Could you check a few things on this model? Use its own coordinates, in mm. A direction names the side the tool comes from. Give positions to 0.01 mm unless a question says otherwise; leave off trailing zeros. Order: outer loops, then holes, each group sorted by start corner. A loop starts at its lowest first (then second) coordinate and runs counter-clockwise, first axis right, second up. Notation, with made-up numbers: M 34,5.25 L 40,5.25 A9 ccw 40,11.25 Z; hole C 43,82.25 d8. An arc over 180 degrees is marked long. Answer in a Markdown table with one row per item. Add a question column.
```python
from build123d import *

# Parameters (mm, degrees)
F0_W         = 4.5
F0_H         = 70
F0_W_2       = 4
F0_H_2       = 34
F1_DEPTH     = 5
F2_W         = 5
F2_H         = 10
F2_W_2       = 4
F2_H_2       = 5.5
F3_DEPTH     = 13
F4_R         = 2.1
F4_R_2       = 1
F5_DEPTH     = 28.001
F6_R         = 2.1
F7_DEPTH     = 3
F8_R         = 3.6
F8_R_2       = 2.1
F9_DEPTH     = 3.8
F10_R        = 7
F11_T1_DEPTH = 5


# Not quite as in the source:
# - a fillet or chamfer that OpenCascade refuses, or shapes differently, is made with other operations: its cross-section is extruded or revolved along the edge and cut away or added


with BuildPart() as f1:
    # F0 (on Front) → F1 (new body)
    with BuildSketch(Plane.XZ):
        Polygon((-8, -44), (8, -44), (8, 44), (-8, 44), (-8, 42), (-8, 8), align=None)
        Rectangle(F0_W, F0_H, mode=Mode.SUBTRACT)
        Polygon((-8, 44), (8, 44), (14, 44), (14, 54), (-14, 54), (-14, 44), align=None)
        with Locations((-10, 25)):
            Rectangle(F0_W_2, F0_H_2)
    extrude(amount=F1_DEPTH)

    # F2 (on face) → F3 (join)
    with BuildSketch(Plane.XZ.offset(5)):
        with Locations((11.5, 49)):
            Rectangle(F2_W, F2_H)
        with Locations((-11.5, 49)):
            Rectangle(F2_W, F2_H)
        with Locations((-10, 10.75)):
            Rectangle(F2_W_2, F2_H_2)
        with Locations((-10, 39.25)):
            Rectangle(F2_W_2, F2_H_2)
    extrude(amount=F3_DEPTH)

    # F4 (on face) → F5 (cut, through all)
    with BuildSketch(Plane(origin=(-14, 0, 0), x_dir=(0, -1, 0), z_dir=(-1, 0, 0))):
        with Locations((13, 49)):
            Circle(F4_R)
        with Locations((15.25, 39.25)):
            Circle(F4_R_2)
        with Locations((15.25, 10.75)):
            Circle(F4_R_2)
    extrude(amount=-F5_DEPTH, mode=Mode.SUBTRACT)

    # F6 (on face) → F7 (cut)
    with BuildSketch(Plane(origin=(-14, 0, 0), x_dir=(0, -1, 0), z_dir=(-1, 0, 0))):
        Polygon((15.0784609691, 45.4), (17.1569219382, 49), (15.0784609691, 52.6), (10.9215390309, 52.6), (8.8430780618, 49), (10.9215390309, 45.4), align=None)
        with Locations((13, 49)):
            Circle(F6_R, mode=Mode.SUBTRACT)
    extrude(amount=-F7_DEPTH, mode=Mode.SUBTRACT)

    # F8 (on face) → F9 (cut)
    with BuildSketch(Plane.YZ.offset(14)):
        with Locations((-13, 49)):
            Circle(F8_R)
        with Locations((-13, 49)):
            Circle(F8_R_2, mode=Mode.SUBTRACT)
    extrude(amount=-F9_DEPTH, mode=Mode.SUBTRACT)

    # F10
    f10_edges = [f1.edges().sort_by_distance(p)[0] for p in [
        (8, -2.5, -44),
        (-8, -2.5, -44),
    ]]
    fillet(f10_edges, radius=F10_R)

    # F11: fillet of radius 2.5 on 4 edges, made by hand

    # F11_s2 → F11_t1 (join)
    with BuildSketch(Plane.XZ):
        with BuildLine():
            ThreePointArc((0.25, -35), (-1.517766953, -34.267766953), (-2.25, -32.5))
            Line((-2.25, -32.5), (-2.25, -35))
            Line((-2.25, -35), (0.25, -35))
        make_face()
        with BuildLine():
            ThreePointArc((2.25, -32.5), (1.517766953, -34.267766953), (-0.25, -35))
            Line((-0.25, -35), (2.25, -35))
            Line((2.25, -35), (2.25, -32.5))
        make_face()
        with BuildLine():
            ThreePointArc((-2.25, 32.5), (-1.517766953, 34.267766953), (0.25, 35))
            Line((0.25, 35), (-2.25, 35))
            Line((-2.25, 35), (-2.25, 32.5))
        make_face()
        with BuildLine():
            ThreePointArc((2.25, 32.5), (1.517766953, 34.267766953), (-0.25, 35))
            Line((-0.25, 35), (2.25, 35))
            Line((2.25, 35), (2.25, 32.5))
        make_face()
    extrude(amount=F11_T1_DEPTH)


solid = f1.part
```
1. Suppose I cut it at C-C on z = 10.75. List the corners of the cut face in (x, y) for me, plus the area to 4 significant figures.
2. Suppose I cut it at D-D on x = 7. List the corners of the cut face in (y, z) for me.
3. If I drill on line 1 along X through (y, z) = (-1.5, 12.5); line 2 along Z through (x, y) = (9.6, -13); line 3 along Z through (x, y) = (11, -14), over which ranges is the centre line in solid material (lowest first)? Write a range as [from, to].
4. Thinking about a two-plate mould opening in Z: for faces 1 (the flat face through (9, -10, 49)), 2 (the cylindrical face through (-1.587, -2.465, -34.196)), 3 (the flat face through (-11, -9, 44)), 4 (the cylindrical face through (-6, -2.5, -41.9)), which applies, pulls with the +Z half, pulls with the -Z half, needs draft (parallel to the pull), parting line crosses it, or undercut?
5. Will these pins go through, and if not, where does the flat tip stop? P1, Ø1, axis at y = -5, z = -0.5, coming from the +X side; P2, Ø1.5, axis at y = -2.5, z = 2, coming from the -X side; P3, Ø4.5, axis at y = -11.5, z = 40, coming from the +X side.
6. Suppose I cut it at B-B on z = 39.25. List the corners of the cut face in (x, y) for me, plus the area to 3 significant figures.
7. Suppose I cut it at A-A on y = -13. Count the separate pieces of the cut face and the enclosed holes in it, plus the area to 3 significant figures.
8. For faces 5 (the flat face through (8, -2, 3)), 6 (the flat face through (-13, -16, 47)), 7 (the flat face through (-8, -11, 39)), which set-ups out of +Z, -Z, +X, -X, +Y, -Y let a thin tool reach every point of the face, with its end or its side?
Findings below:
| question | item | result |
|---|---|---|
| 1 | outline | M -12,-18 L -8,-18 L -8,-16.25 L -12,-16.25 Z; M -12,-14.25 L -8,-14.25 L -8,-5 L -2.25,-5 L -2.25,0 L -12,0 Z; M 2.25,-5 L 8,-5 L 8,0 L 2.25,0 Z |
| 1 | area | 121.5 mm2 |
| 2 | outline | M -5,-40.61 L 0,-40.61 L 0,54 L -5,54 Z |
| 3 | line 1 | [-12, -2.25], [2.25, 8] |
| 3 | line 2 | [44, 46.9], [51.1, 54] |
| 3 | line 3 | [44, 45.54], [52.46, 54] |
| 4 | face 1 | needs draft |
| 4 | face 2 | undercut |
| 4 | face 3 | undercut |
| 4 | face 4 | pulls with the -Z half |
| 5 | P1 | x = 8 |
| 5 | P2 | x = -8 |
| 5 | P3 | x = -8 |
| 6 | outline | M -12,-18 L -8,-18 L -8,-16.25 L -12,-16.25 Z; M -12,-14.25 L -8,-14.25 L -8,-5 L 8,-5 L 8,0 L -12,0 Z |
| 6 | area | 144 mm2 |
| 7 | separate pieces | 6 |
| 7 | enclosed holes | 0 |
| 7 | area | 81.6 mm2 |
| 8 | face 5 | -Z, +X, +Y, -Y |
| 8 | face 6 | -X |
| 8 | face 7 | +Z, -Z, +X, -Y |
